```python
from build123d import *

# Parameters (mm, degrees)
SKETCH3_R           = 3.2385
BOSS_EXTRUDE1_DEPTH = 63.5
FILLET1_R           = 0.254


with BuildPart() as part:
    # Sketch3 → Boss-Extrude1 (new body, symmetric)
    with BuildSketch(Plane.XY):
        with BuildLine():
            Line((-11.049, 12.7), (-3.302, 12.7))
            Line((-3.302, 12.7), (-3.302, 10.328863887))
            Line((-3.302, 10.328863887), (-6.985, 10.328863887))
            ThreePointArc((-6.985, 10.328863887), (-7.454330803, 10.01526707), (-7.344210245, 9.461653642))
            Line((-7.344210245, 9.461653642), (-3.452505379, 5.569948776))
            ThreePointArc((-3.452505379, 5.569948776), (-2.628470073, 5.019345987), (-1.656454155, 4.826))
            Line((-1.656454155, 4.826), (1.656454155, 4.826))
            ThreePointArc((1.656454155, 4.826), (2.628470073, 5.019345987), (3.452505379, 5.569948776))
            Line((3.452505379, 5.569948776), (7.344210245, 9.461653642))
            ThreePointArc((7.344210245, 9.461653642), (7.454330803, 10.01526707), (6.985, 10.328863887))
            Line((6.985, 10.328863887), (3.302, 10.328863887))
            Line((3.302, 10.328863887), (3.302, 12.7))
            Line((3.302, 12.7), (11.049, 12.7))
            ThreePointArc((11.049, 12.7), (12.216433296, 12.216433296), (12.7, 11.049))
            Line((12.7, 11.049), (12.7, 1.651))
            ThreePointArc((12.7, 1.651), (12.216433296, 0.483566704), (11.049, 0))
            Line((11.049, 0), (-11.049, 0))
            ThreePointArc((-11.049, 0), (-12.216433296, 0.483566704), (-12.7, 1.651))
            Line((-12.7, 1.651), (-12.7, 11.049))
            ThreePointArc((-12.7, 11.049), (-12.216433296, 12.216433296), (-11.049, 12.7))
        make_face()
        with Locations((8.509, 4.064)):
            Circle(SKETCH3_R, mode=Mode.SUBTRACT)
        with Locations((-8.509, 4.064)):
            Circle(SKETCH3_R, mode=Mode.SUBTRACT)
    extrude(amount=BOSS_EXTRUDE1_DEPTH, both=True)

    # Fillet1
    fillet1_edges = [part.edges().sort_by_distance(p)[0] for p in [
        (-3.302, 12.7, 0),
        (-3.302, 10.328863887, 0),
        (3.302, 10.328863887, 0),
        (3.302, 12.7, 0),
    ]]
    fillet(fillet1_edges, radius=FILLET1_R)


solid = part.part
```
Part model, mm, in its own coordinate system. A direction names the side the tool comes from. Round coordinates to 2 decimals unless told otherwise and drop trailing zeros. Loops run counter-clockwise (first coordinate to the right, second up) from the corner with the lowest first, then second, coordinate; pieces in that order, holes last. Notation, with made-up numbers: (48.25, 21.25) -> (89.25, 21.25) arc R23 cw to (89.25, 35.25) -> close; hole circle Ø11 at (-39, -34.75). An arc over 180 degrees is marked (long way). Use a Markdown table: item, result.
1) Cut at B-B, the plane x = -0.25. List the corners of the cut face in (y, z), and give its area (3 significant figures).
The answers:
| item | result |
|---|---|
| outline | (0, -63.5) -> (4.83, -63.5) -> (4.83, 63.5) -> (0, 63.5) -> close |
| area | 613 mm2 |
2) Cut at A-A, the plane z = -34. State how many separate pieces and enclosed holes the cut face has, and give its area (3 significant figures).
The answers:
| item | result |
|---|---|
| separate pieces | 1 |
| enclosed holes | 2 |
| area | 179 mm2 |
3) Probe line 1 (Y direction, x = -7.25, z = 2); line 2 (X direction, y = 6.25, z = 41); line 3 (X direction, y = 2, z = 45). List the from-to ranges inside material, lowest first. Write a range as [from, to].
The answers:
| item | result |
|---|---|
| line 1 | y = [0, 1.08], [7.05, 9.37], [10.25, 12.7] |
| line 2 | x = [-12.7, -10.9], [-6.12, -4.13], [4.13, 6.12], [10.9, 12.7] |
| line 3 | x = [-12.7, -11], [-6.01, 6.01], [11, 12.7] |
4) Drop flat-ended pins along their axis: pin 1 Ø5 at (x, y) = (-8.509, 4.064) entering from -Z; pin 2 Ø0.9 at (y, z) = (12, 20.5) entering from +X; pin 3 Ø2.5 at (x, z) = (-0.5, -13) entering from +Y. Give the stop position or say it passes through.
The answers:
| item | result |
|---|---|
| pin 1 | passes through |
| pin 2 | stops at x = 12.62 |
| pin 3 | stops at y = 4.83 |
5) Pull direction Y, two halves, no side cores. Call faces 4 (the flat face through (-7, 12.7, 1)), 5 (the cylindrical face through (11.598, 5.037, -0.889)), 6 (the flat face through (0, 0, 1)), 7 (the flat face through (-12.7, 6, 1)): pulls with the +Y half, pulls with the -Y half, needs draft (parallel to the pull), parting line crosses it, or undercut.
The answers:
| item | result |
|---|---|
| face 4 | pulls with the +Y half |
| face 5 | undercut |
| face 6 | pulls with the -Y half |
| face 7 | needs draft |
6) Tool access for faces 1 (the flat face through (-5, 10.329, 1)), 2 (the flat face through (0, 4, 63.5)), 3 (the flat face through (0, 4.826, 1)): list every direction of +Z, -Z, +X, -X, +Y, -Y with a clear straight run to the whole face (end or side of a thin tool).
The answers:
| item | result |
|---|---|
| face 1 | +Z, -Z |
| face 2 | +Z, +X, -X, +Y, -Y |
| face 3 | +Z, -Z, +Y |
